Source: CAD feature listing. Evaluate the final solid. Frame: model axes, mm. Give positions to 0.01 mm unless a question says otherwise; leave off trailing zeros. Loops run counter-clockwise (first coordinate to the right, second up) from the corner with the lowest first, then second, coordinate; pieces in that order, holes last. Notation, with made-up numbers: (0, 64) - (20, 64) arc R15 ccw to (20, 76) - close; hole circle Ø7 at (66.5, -17). An arc over 180 degrees is marked (long way). Put each result on its own line as item: value.
```python
from build123d import *

# Parameters (mm, degrees)
SKETCH_1_W      = 197
SKETCH_1_H      = 20.5
EXTRUDE_1_DEPTH = 3
HOLE_WIZARD_1_D = 3.5
HOLE_WIZARD_2_D = 3.5


with BuildPart() as part:
    # 草图1 → 凸台-拉伸1 (new body)
    with BuildSketch(Plane(origin=(0, 0, 0), x_dir=(1, 0, 0), z_dir=(0, 1, 0))):
        with Locations((98.5, 10.25)):
            Rectangle(SKETCH_1_W, SKETCH_1_H)
    extrude(amount=EXTRUDE_1_DEPTH)

    # 孔1 (through all)
    with Locations(Plane(origin=(0, 3, 0), x_dir=(1, 0, 0), z_dir=(0, 1, 0))):
        with Locations((8, 5), (189, 5)):
            Hole(HOLE_WIZARD_1_D / 2)

    # 孔2 (through all)
    with Locations(Plane(origin=(0, 3, 0), x_dir=(1, 0, 0), z_dir=(0, 1, 0))):
        with Locations((98.5, 15.5), (141.25, 15.5), (55.75, 15.5), (13, 15.5), (184, 15.5)):
            Hole(HOLE_WIZARD_2_D / 2)


solid = part.part
```
1) Section query A-A, the plane z = -5. Output: boundary loops of the cut face in (x, y).
Check result:
outline: (0, 0) - (6.25, 0) - (6.25, 3) - (0, 3) - close; (9.75, 0) - (187.25, 0) - (187.25, 3) - (9.75, 3) - close; (190.75, 0) - (197, 0) - (197, 3) - (190.75, 3) - close
2) Section query B-B, the plane y = 1.65. Output: boundary loops of the cut face in (x, z), plus the area to 3 significant figures.
Check result:
outline: (0, -20.5) - (197, -20.5) - (197, 0) - (0, 0) - close; hole circle Ø3.5 at (8, -5); hole circle Ø3.5 at (13, -15.5); hole circle Ø3.5 at (55.75, -15.5); hole circle Ø3.5 at (98.5, -15.5); hole circle Ø3.5 at (141.25, -15.5); hole circle Ø3.5 at (184, -15.5); hole circle Ø3.5 at (189, -5)
area: 3,970 mm²
3) Section query D-D, the plane z = -15.5. Output: boundary loops of the cut face in (x, y), plus the area to 4 significant figures.
Check result:
outline: (0, 0) - (11.25, 0) - (11.25, 3) - (0, 3) - close; (14.75, 0) - (54, 0) - (54, 3) - (14.75, 3) - close; (57.5, 0) - (96.75, 0) - (96.75, 3) - (57.5, 3) - close; (100.25, 0) - (139.5, 0) - (139.5, 3) - (100.25, 3) - close; (143, 0) - (182.25, 0) - (182.25, 3) - (143, 3) - close; (185.75, 0) - (197, 0) - (197, 3) - (185.75, 3) - close
area: 538.5 mm²
4) Section query C-C, the plane x = 8. Output: boundary loops of the cut face in (y, z), plus the area to 3 significant figures.
Check result:
outline: (0, -20.5) - (3, -20.5) - (3, -6.75) - (0, -6.75) - close; (0, -3.25) - (3, -3.25) - (3, 0) - (0, 0) - close
area: 51.0 mm²
5) Mould query, pull axis Z, two halves, no side actions, for faces 1 (the flat face through (197, 1, -10)), 2 (the cylindrical face through (187.331, 1.479, -5.526)), 3 (the flat face through (97, 1, 0)), 4 (the cylindrical face through (54.081, 1.479, -16.026)). Classes: pulls with the +Z half, pulls with the -Z half, needs draft (parallel to the pull), parting line crosses it, or undercut.
Check result:
face 1: needs draft
face 2: undercut
face 3: pulls with the +Z half
face 4: undercut
6) Material intervals for line 1 along X through (y, z) = (1.05, -15.5); line 2 along Z through (x, y) = (184, 1.4); line 3 along X through (y, z) = (2.05, -14.75), sorted ascending. Write a range as [from, to].
Check result:
line 1: [0, 11.25], [14.75, 54], [57.5, 96.75], [100.25, 139.5], [143, 182.25], [185.75, 197]
line 2: [-20.5, -17.25], [-13.75, 0]
line 3: [0, 11.42], [14.58, 54.17], [57.33, 96.92], [100.08, 139.67], [142.83, 182.42], [185.58, 197]
7) Pin query (flat end, axial travel): P1, Ø1, axis at y = 2.5, z = -15.5, coming from the -X side; P2, Ø3, axis at x = 8, z = -5, coming from the -Y side. Return the tip coordinate at first contact, or that it passes through.
Check result:
P1: x = 0
P2: through
